Here's how the part is built. I have some questions about the finished solid (model axes, mm). Face numbers are marked on the shaded views. A direction names the side the tool comes from. Coordinates: 2 decimals unless noted, no trailing zeros. Loops run counter-clockwise (first coordinate to the right, second up) from the corner with the lowest first, then second, coordinate; pieces in that order, holes last. Notation, with made-up numbers: M 77,78 L 110,78 A14 ccw 110,95 Z; hole C -5,-10.5 d10. An arc over 180 degrees is marked long. Use CSV: the item, a comma, the result in double quotes. Start each with the question number.
Q1. Please list where these lines run through material, in increasing order: probe 1 along X at (y, z) = (-11, 2); probe 2 along Z at (x, y) = (83, -34.5); probe 3 along X at (y, z) = (-26, -2.75). Write a range as [from, to].
Q2. Which directions (+Z, -Z, +X, -X, +Y, -Y) give clear straight access to the entire face, cutting with the end or side of a thin tool? Please do the marked faces 1, 2 and 3.
Q3. If we section it at C-C (y = -71.5): Please give me the cut outline in (x, z).
Q4. If we section it at A-A (z = 3.5): Please give me the cut outline in (x, y).
Q5. For pin 1 Ø6 at (x, y) = (40, -64.5) entering from +Z; pin 2 Ø4 at (x, y) = (63, -51.5) entering from -Z, each with a flat end and sliding along its axis, tell me the tip position at first contact or that it passes through.
Q6. If we section it at B-B (x = 82): Please give me the cut outline in (y, z), and give its area (3 significant figures).
Q7. If we section it at D-D (z = -1.5): Please give me the cut outline in (x, y), and give its area (3 significant figures).
from build123d import *

# Parameters (mm, degrees)
SKETCH_1_W      = 80
SKETCH_1_H      = 80
EXTRUDE_1_DEPTH = 5
SKETCH_2_W      = 4
SKETCH_2_H      = 80
EXTRUDE_2_DEPTH = 4
SKETCH_2_2_W    = 4
SKETCH_2_2_H    = 80
EXTRUDE_3_DEPTH = 12
SKETCH_3_W      = 4
SKETCH_3_H      = 80
EXTRUDE_4_DEPTH = 9
SKETCH_6_W      = 8
SKETCH_6_H      = 5
EXTRUDE_5_DEPTH = 80


with BuildPart() as part:
    # 草图1 → 凸台-拉伸1 (new body)
    with BuildSketch(Plane.XY):
        with Locations((40, -40)):
            Rectangle(SKETCH_1_W, SKETCH_1_H)
    extrude(amount=EXTRUDE_1_DEPTH)

    # 草图2 → 凸台-拉伸2 (add)
    with BuildSketch(Plane(origin=(80, 0, 0), x_dir=(0, 0, -1), z_dir=(1, 0, 0))):
        with Locations((-7, -40)):
            Rectangle(SKETCH_2_W, SKETCH_2_H)
        with Locations((2, -40)):
            Rectangle(SKETCH_2_W, SKETCH_2_H)
    extrude(amount=-EXTRUDE_2_DEPTH)

    # 草图2<2> → 凸台-拉伸3 (add)
    with BuildSketch(Plane(origin=(80, 0, 0), x_dir=(0, 0, -1), z_dir=(1, 0, 0))):
        with Locations((-7, -40)):
            Rectangle(SKETCH_2_2_W, SKETCH_2_2_H)
        with Locations((2, -40)):
            Rectangle(SKETCH_2_2_W, SKETCH_2_2_H)
    extrude(amount=EXTRUDE_3_DEPTH)

    # 草图3 → 凸台-拉伸4 (add)
    with BuildSketch(Plane.XY.offset(9)):
        with Locations((90, -40)):
            Rectangle(SKETCH_3_W, SKETCH_3_H)
    extrude(amount=-EXTRUDE_4_DEPTH)

    # 草图6 → 凸台-拉伸5 (add)
    with BuildSketch(Plane.XZ.offset(80)):
        Polygon((-16, -4), (0, -4), (0, 0), (0, 5), (0, 9), (-16, 9), align=None)
        with Locations((-8, 2.5)):
            Rectangle(SKETCH_6_W, SKETCH_6_H, mode=Mode.SUBTRACT)
    extrude(amount=-EXTRUDE_5_DEPTH)


solid = part.part
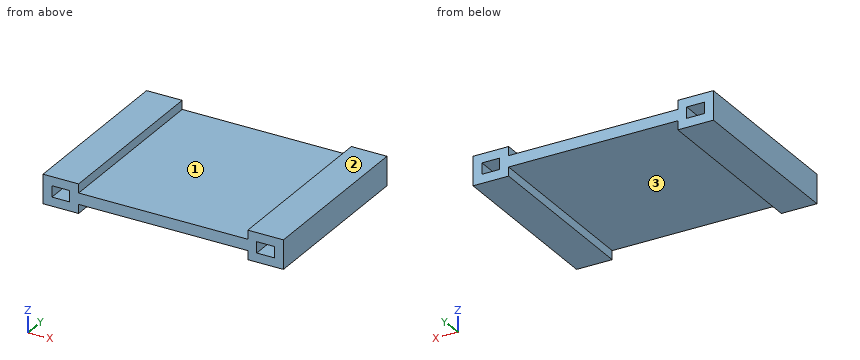
Results below:
1,probe 1,"[-16, -12], [-4, 80], [88, 92]"
1,probe 2,"[-4, 0], [5, 9]"
1,probe 3,"[-16, 0], [76, 92]"
2,face 1,"+Z, +Y, -Y"
2,face 2,"+Z, +X, -X, +Y, -Y"
2,face 3,"-Z, +Y, -Y"
3,outline,"M -16,-4 L 0,-4 L 0,0 L 76,0 L 76,-4 L 92,-4 L 92,9 L 76,9 L 76,5 L 0,5 L 0,9 L -16,9 Z; hole M -12,0 L -4,0 L -4,5 L -12,5 Z; hole M 80,0 L 88,0 L 88,5 L 80,5 Z"
4,outline,"M -16,-80 L -12,-80 L -12,0 L -16,0 Z; M -4,-80 L 80,-80 L 80,0 L -4,0 Z; M 88,-80 L 92,-80 L 92,0 L 88,0 Z"
5,pin 1,"z = 5"
5,pin 2,"z = 0"
6,outline,"M -80,-4 L 0,-4 L 0,0 L -80,0 Z; M -80,5 L 0,5 L 0,9 L -80,9 Z"
6,area,"640 mm^2"
7,outline,"M -16,-80 L 0,-80 L 0,0 L -16,0 Z; M 76,-80 L 92,-80 L 92,0 L 76,0 Z"
7,area,"2,560 mm^2"
